Verification items for the finished model (mm, model axes). A direction names the side the tool comes from. Coordinates: 2 decimals unless noted, no trailing zeros. Order: outer loops, then holes, each group sorted by start corner. A loop starts at its lowest first (then second) coordinate and runs counter-clockwise, first axis right, second up. Notation, with made-up numbers: M 87.25,-36 L 141.25,-36 A21 cw 141.25,-15 Z; hole C 50.25,-7 d2. An arc over 180 degrees is marked long. Return JSON: item names as keys, results as strings. Group by question number.
Q1. Mould release check, pull along Z, two halves, no side actions. Record for faces 6 (the face through (4.575, -9, 7)), 7 (the face through (0.1, -9.19, 8.67)), 8 (the face through (-7, 9, 2)): pulls with the +Z half, pulls with the -Z half, needs draft (parallel to the pull), parting line crosses it, or undercut.
Q2. Go/stop test with flat-tipped pins: pin 1 Ø3 at (x, z) = (1, 7.5) entering from +Y; pin 2 Ø7 at (x, y) = (-8.5, 10) entering from +Z; pin 3 Ø2 at (y, z) = (5, 6.5) entering from +X. Record where each tip stops, or that it passes through.
Q3. Section check D-D, the plane x = -9. Enter the section's corners in (y, z), then the cut area to 3 significant figures.
Q4. Access from +Z, -Z, +X, -X, +Y, -Y to the whole of each face (thin tool, end or side, straight path). Record for faces 1 (the face through (-5.425, 26, 1)), 2 (the face through (4.602, -2, 5)), 3 (the face through (-3.398, -2, 5)), 4 (the face through (11, 14.042, 1)), 5 (the face through (-5.398, -1, 6)).
Q5. Thickness scan on probe 1 along X at (y, z) = (-4, 9.5); probe 2 along Y at (x, z) = (2.5, 4.25); probe 3 along Z at (x, y) = (5, -3.5). Record the ranges inside material, lowest first.
Q6. Section check B-B, the plane z = 1.5. Enter the section's corners in (x, y), then the cut area to 3 significant figures.
Q7. Section check C-C, the plane y = 25.5. Enter the section's corners in (x, z), then the cut area to 3 significant figures.
from build123d import *

# Parameters (mm, degrees)
ESBO_O1_R                = 1
RESSALTO_EXTRUS_O1_DEPTH = 2
ESBO_O2_W                = 35
ESBO_O2_H                = 2
RESSALTO_EXTRUS_O2_DEPTH = 10
ESBO_O3_R                = 1.75
CORTE_EXTRUS_O1_DEPTH    = 10
ESBO_O4_W                = 12.527176897
ESBO_O4_H                = 10
ESBO_O4_W_2              = 12.5
CORTE_EXTRUS_O2_DEPTH    = 10
RESSALTO_EXTRUS_O3_DEPTH = 10
ESBO_O6_W                = 6
ESBO_O6_H                = 22.25
CORTE_EXTRUS_O3_DEPTH    = 10


with BuildPart() as part:
    # Esboço1 → Ressalto-extrusão1 (new body)
    with BuildSketch(Plane.XY):
        Polygon((-17.925350174, 14.041666667), (-5.425350174, 14.041666667), (-5.425350174, 38.291666667), (4.574649826, 38.291666667), (4.574649826, 14.041666667), (17.074649826, 14.041666667), (17.074649826, -10.208333333), (-17.925350174, -10.208333333), align=None)
        with Locations((-0.425350174, 32.541666667)):
            Circle(ESBO_O1_R, mode=Mode.SUBTRACT)
        with Locations((-0.425350174, -4.458333333)):
            Circle(ESBO_O1_R, mode=Mode.SUBTRACT)
    extrude(amount=RESSALTO_EXTRUS_O1_DEPTH)

    # Esboço2 → Ressalto-extrusão2 (add)
    with BuildSketch(Plane.XY.offset(2)):
        with Locations((-0.425350174, -9.208333333)):
            Rectangle(ESBO_O2_W, ESBO_O2_H)
    extrude(amount=RESSALTO_EXTRUS_O2_DEPTH)

    # Esboço3 → Corte-extrusão1 (cut)
    with BuildSketch(Plane(origin=(0, -8.208333333, 0), x_dir=(1, 0, 0), z_dir=(0, 1, 0))):
        with Locations(Location((-0.425350174, -7, 0), (0, 0, 270))):
            Circle(ESBO_O3_R)
    extrude(amount=-CORTE_EXTRUS_O1_DEPTH, mode=Mode.SUBTRACT)

    # Esboço4 → Corte-extrusão2 (cut)
    with BuildSketch(Plane(origin=(0, -8.208333333, 0), x_dir=(1, 0, 0), z_dir=(0, 1, 0))):
        with Locations((-11.661761726, -7)):
            Rectangle(ESBO_O4_W, ESBO_O4_H)
        with Locations((10.824649826, -7)):
            Rectangle(ESBO_O4_W_2, ESBO_O4_H)
    extrude(amount=-CORTE_EXTRUS_O2_DEPTH, mode=Mode.SUBTRACT)

    # Esboço5 → Ressalto-extrusão3 (add)
    with BuildSketch(Plane.ZY.offset(5.398173277)):
        Polygon((12, -8.208333333), (2, 14.041666667), (2, -8.208333333), align=None)
    extrude(amount=-RESSALTO_EXTRUS_O3_DEPTH)

    # Esboço6 → Corte-extrusão3 (cut)
    with BuildSketch(Plane.XY.offset(12)):
        with Locations((-0.398173277, 2.916666667)):
            Rectangle(ESBO_O6_W, ESBO_O6_H)
    extrude(amount=-CORTE_EXTRUS_O3_DEPTH, mode=Mode.SUBTRACT)


solid = part.part
Numbers:
{
 "1": {"face 6": "needs draft", "face 7": "undercut", "face 8": "pulls with the +Z half"},
 "2": {"pin 1": "stops at y = -8.21", "pin 2": "stops at z = 4.55", "pin 3": "stops at x = 4.6"},
 "3": {"outline": "M -10.21,0 L 14.04,0 L 14.04,2 L -10.21,2 Z", "area": "48.5 mm2"},
 "4": {"face 1": "+Z, -Z, -X, +Y", "face 2": "+Z, +X, +Y, -Y", "face 3": "+Z, +Y", "face 4": "+Z, -Z, +X, +Y", "face 5": "+Z, -X, +Y, -Y"},
 "5": {"probe 1": "x = -5.4 to -3.4, 2.6 to 4.6", "probe 2": "y = -10.21 to -8.21", "probe 3": "z = 0 to 2"},
 "6": {"outline": "M -17.93,-10.21 L 17.07,-10.21 L 17.07,14.04 L 4.57,14.04 L 4.57,38.29 L -5.43,38.29 L -5.43,14.04 L -17.93,14.04 Z; hole C -0.43,-4.46 d2; hole C -0.43,32.54 d2", "area": "1,080 mm2"},
 "7": {"outline": "M -5.43,0 L 4.57,0 L 4.57,2 L -5.43,2 Z", "area": "20.0 mm2"}
}
